Source: CAD feature listing. Evaluate the final solid. Frame: model axes, mm. Face numbers are marked on the shaded views. A direction names the side the tool comes from. Give positions to 0.01 mm unless a question says otherwise; leave off trailing zeros. Loops run counter-clockwise (first coordinate to the right, second up) from the corner with the lowest first, then second, coordinate; pieces in that order, holes last. Notation, with made-up numbers: (30, 11.25) - (53, 11.25) arc R30 cw to (53, 50.25) - close; hole circle Ø2 at (3, 15). An arc over 180 degrees is marked (long way). Write each question's results on one line, items separated by ' | '. Start each with the question number.
(1) Cut plane D-D on x = 28. Return the cut outline in (y, z), then the cut area to 3 significant figures.
(2) Contact query for flat-ended pins moving along their axis: pin 1 (10 mm diameter, centred on y = -17, z = 23.5, fed in from +X); pin 2 (1.5 mm diameter, centred on x = 25.5, z = 17.5, fed in from -Y); pin 3 (7 mm diameter, centred on x = 0, y = 0, fed in from +Z); pin 4 (6 mm diameter, centred on x = 14.5, y = -25, fed in from -Z). Output: stop coordinate, or through.
(3) Material intervals for line 1 along Y through (x, z) = (0, 22.5); line 2 along Z through (x, y) = (27, 15); line 3 along Y through (x, z) = (0, 10), sorted ascending. Write a range as [from, to].
(4) Reachability of the marked faces 1 and 2 from +Z, -Z, +X, -X, +Y, -Y: full face, straight path, thin tool, end or side. Return the list, or none.
(5) Cut plane C-C on z = 14. Return the cut outline in (x, y).
(6) Cut plane A-A on x = 0. Return the cut outline in (y, z).
(7) Pull-direction query (Z, two-part tool) for the marked faces 3, 4 and 5; classes: pulls with the +Z half, pulls with the -Z half, needs draft (parallel to the pull), parting line crosses it, or undercut.
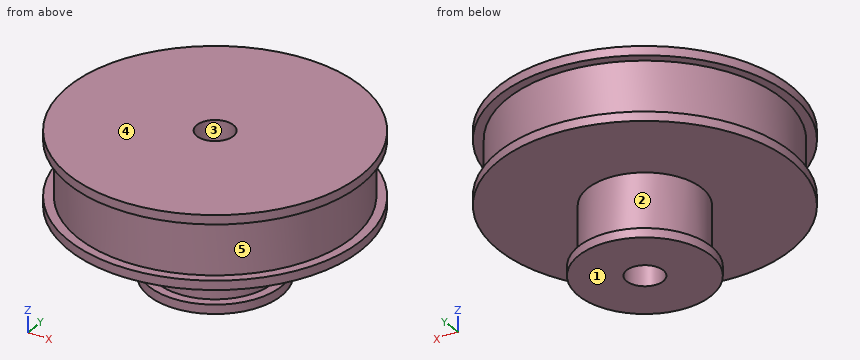
from build123d import *

# Parameters (mm, degrees)
SKETCH_1_R          = 12.5
EXTRUDE_1_DEPTH     = 15
SKETCH_2_R          = 30
EXTRUDE_2_DEPTH     = 14
SKETCH_3_R          = 32
EXTRUDE_3_DEPTH     = 2
SKETCH_4_R          = 32
EXTRUDE_4_DEPTH     = 2
SKETCH_5_R          = 14.5
EXTRUDE_5_DEPTH     = 2
SKETCH_6_R          = 4
CUT_EXTRUDE_1_DEPTH = 55.854352608


with BuildPart() as part:
    # 草图1 → 拉伸1 (new body)
    with BuildSketch(Plane.XY):
        Circle(SKETCH_1_R)
    extrude(amount=EXTRUDE_1_DEPTH)

    # 草图2 → 拉伸2 (add)
    with BuildSketch(Plane.XY.offset(15)):
        Circle(SKETCH_2_R)
    extrude(amount=EXTRUDE_2_DEPTH)

    # 草图3 → 拉伸3 (add)
    with BuildSketch(Plane.XY.offset(29)):
        Circle(SKETCH_3_R)
    extrude(amount=-EXTRUDE_3_DEPTH)

    # 草图4 → 拉伸4 (add)
    with BuildSketch(Plane(origin=(0, 0, 15), x_dir=(-1, 0, 0), z_dir=(0, 0, -1))):
        with Locations(Location((0, 0, 0), (0, 0, 180))):
            Circle(SKETCH_4_R)
    extrude(amount=EXTRUDE_4_DEPTH)

    # 草图5 → 拉伸5 (add)
    with BuildSketch(Plane(origin=(0, 0, 0), x_dir=(-1, 0, 0), z_dir=(0, 0, -1))):
        Circle(SKETCH_5_R)
    extrude(amount=EXTRUDE_5_DEPTH)

    # 草图6 → 切除-拉伸1 (cut, through all)
    with BuildSketch(Plane.XY.offset(29)):
        Circle(SKETCH_6_R)
    extrude(amount=-CUT_EXTRUDE_1_DEPTH, mode=Mode.SUBTRACT)


solid = part.part
Ans:
1) outline: (-15.49, 13) - (15.49, 13) - (15.49, 15) - (10.77, 15) - (10.77, 27) - (15.49, 27) - (15.49, 29) - (-15.49, 29) - (-15.49, 27) - (-10.77, 27) - (-10.77, 15) - (-15.49, 15) - close | area: 382 mm^2
2) pin 1: x = 29.05 | pin 2: y = -16.95 | pin 3: through | pin 4: z = 13
3) line 1: [-30, -4], [4, 30] | line 2: [13, 15], [27, 29] | line 3: [-12.5, -4], [4, 12.5]
4) face 1: -Z, +X, -X, +Y, -Y | face 2: none
5) outline: circle Ø64 at (0, 0); hole circle Ø8 at (0, 0)
6) outline: (-32, 13) - (-12.5, 13) - (-12.5, 0) - (-14.5, 0) - (-14.5, -2) - (-4, -2) - (-4, 29) - (-32, 29) - (-32, 27) - (-30, 27) - (-30, 15) - (-32, 15) - close; (4, -2) - (14.5, -2) - (14.5, 0) - (12.5, 0) - (12.5, 13) - (32, 13) - (32, 15) - (30, 15) - (30, 27) - (32, 27) - (32, 29) - (4, 29) - close
7) face 3: needs draft | face 4: pulls with the +Z half | face 5: undercut
